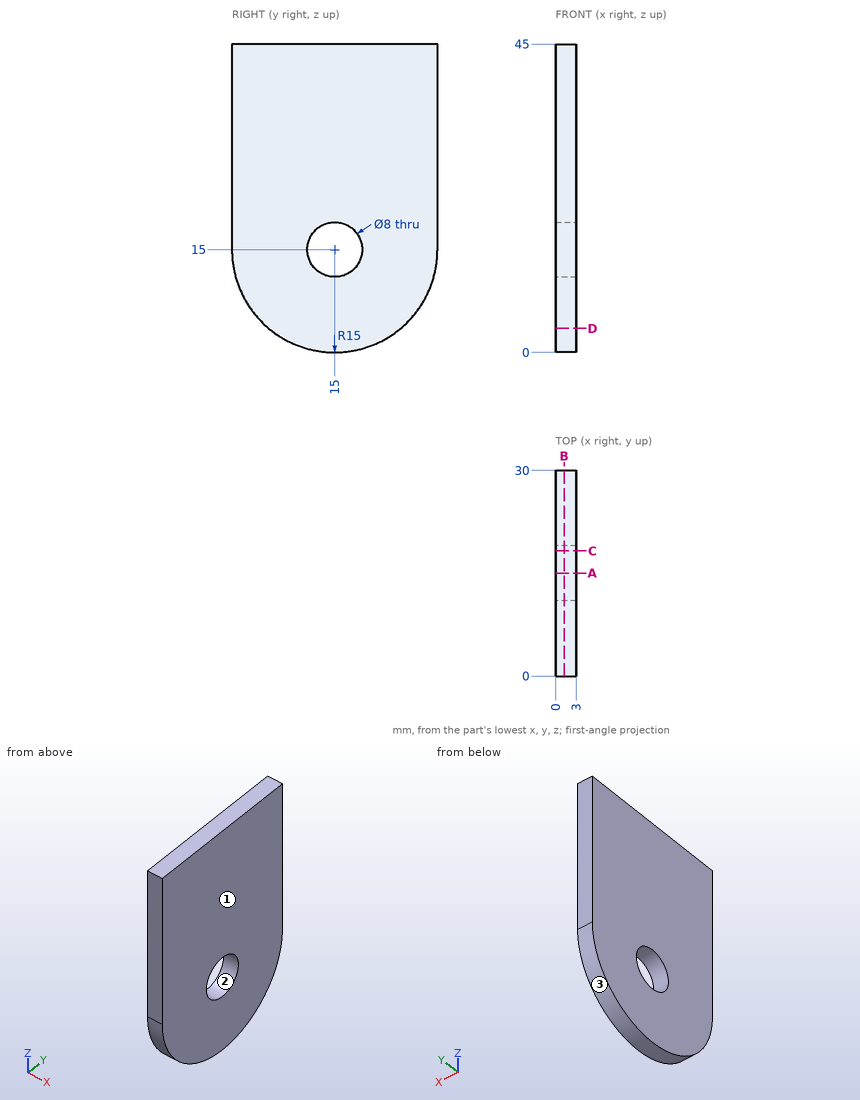
Part print with two shaded views. Sizes in mm from the minimum x, y, z corner. Coordinates: 2 decimals unless noted, no trailing zeros. Write each loop counter-clockwise with the first axis right and the second up, starting at its lowest first coordinate (ties: lowest second). Pieces come first, ordered by that corner, then holes.
(1) Drill centre lines: line 1 (Y direction, x = 0.9, z = 15); line 2 (Y direction, x = 2.7, z = 2); line 3 (Z direction, x = 0.4, y = 6.75). Where is each one in solid material? Low to high.
(2) Cut at B-B on x = 1.25. List the corners of the cut face in (y, z), and give its area (3 significant figures).
(3) Cut at A-A on y = 15. List the corners of the cut face in (x, z).
(4) Cut at C-C on y = 18.25. List the corners of the cut face in (x, z).
(5) Cut at D-D on z = 3.5. List the corners of the cut face in (x, y), and give its area (3 significant figures).
(6) Mould opens along Z. For the marked faces 1, 2 and 3 say: pulls with the +Z half, pulls with the -Z half, needs draft (parallel to the pull), parting line crosses it, or undercut.
Working result:
1. line 1: y = 0 to 11, 19 to 30
1. line 2: y = 7.52 to 22.48
1. line 3: z = 2.47 to 45
2. outline: (0, 15) arc R15 ccw to (30, 15) - (30, 45) - (0, 45) - close; hole circle Ø8 at (15, 15)
2. area: 1,200 mm2
3. outline: (0, 0) - (3, 0) - (3, 11) - (0, 11) - close; (0, 19) - (3, 19) - (3, 45) - (0, 45) - close
4. outline: (0, 0.36) - (3, 0.36) - (3, 12.67) - (0, 12.67) - close; (0, 17.33) - (3, 17.33) - (3, 45) - (0, 45) - close
5. outline: (0, 5.37) - (3, 5.37) - (3, 24.63) - (0, 24.63) - close
5. area: 57.8 mm2
6. face 1: needs draft
6. face 2: undercut
6. face 3: pulls with the -Z half
